Could you check a few things on this model? Use its own coordinates, in mm. Give positions to 0.01 mm unless a question says otherwise; leave off trailing zeros. Loops run counter-clockwise (first coordinate to the right, second up) from the corner with the lowest first, then second, coordinate; pieces in that order, holes last.
1. Imagine slicing it at A-A (x = 0). List the corners of the cut face in (y, z) for me (3 decimals).
2. I need wall thicknesses on line 1 along X through (y, z) = (1.75, -21.5); line 2 along Z through (x, y) = (0, 2.9) (3 decimals); line 3 along Z through (x, y) = (11, 2). Which ranges of each line are inside material? Lowest first, please.
3. Thinking about a two-plate mould opening in Z: for faces 1 (the flat face through (0, 3.81, 14)), 2 (the cylindrical face through (-25.7, 2.425, 19.706)), 3 (the cylindrical face through (14.264, 1.932, -19.645)), which applies, +Z half, -Z half, draft (parallel to the pull), parting line (faces both ways), or undercut?
4. For P1, Ø15.5, axis at x = 0, z = 0, coming from the +Y side; P2, Ø1, axis at x = -1.5, y = 0.5, coming from the -Z side; P3, Ø1, axis at y = 3.5, z = 12.5, coming from the -X side; P4, Ø1.5, axis at x = -8, y = 3, coming from the +Z side, each with a flat end and sliding along its axis, tell me the tip position at first contact or that it passes through.
5. Imagine slicing it at B-B (z = 0). List the corners of the cut face in (x, y) for me (3 decimals).
6. Imagine slicing it at C-C (y = 3.15). List the corners of the cut face in (x, z) for me (1 decimal), plus the area to 3 significant figures.
```python
from build123d import *

# Parameters (mm, degrees)
SKETCH1_W                      = 32.385
SKETCH1_H                      = 3.81
F_7_0_201_DIAMETER_HOLE1_D     = 5.1054
F_7_0_201_DIAMETER_HOLE1_DEPTH = 3.81
HOLE1_D                        = 25.654
HOLE1_DEPTH                    = 3.81
FILLET1_R                      = 1


with BuildPart() as part:
    # Sketch1 → Revolve1 (revolve)
    with BuildSketch(Plane(origin=(0, 0, 0), x_dir=(-1, 0, 0), z_dir=(0, 0, -1))):
        with Locations((-16.1925, 1.905)):
            Rectangle(SKETCH1_W, SKETCH1_H)
    revolve(axis=Axis((0, 0, 0), (0, 1, 0)))

    # #7 (0.201) Diameter Hole1
    with Locations(Plane(origin=(0, 0, 0), x_dir=(-1, 0, 0), z_dir=(0, -1, 0))):
        with Locations((11.90625, 20.622229928), (-11.90625, 20.622229928), (-23.8125, 0), (-11.90625, -20.622229928), (11.90625, -20.622229928), (23.8125, 0)):
            Hole(F_7_0_201_DIAMETER_HOLE1_D / 2, depth=F_7_0_201_DIAMETER_HOLE1_DEPTH)

    # Hole1
    with Locations(Plane(origin=(0, 0, 0), x_dir=(-1, 0, 0), z_dir=(0, -1, 0))):
        with Locations((0, 0)):
            Hole(HOLE1_D / 2, depth=HOLE1_DEPTH)

    # Fillet1
    fillet1_edges = [part.edges().sort_by_distance(p)[0] for p in [
        (-32.385, 0, 0),
    ]]
    fillet(fillet1_edges, radius=FILLET1_R)


solid = part.part
```
Derived:
1. outline: (0, -31.385) arc R1 ccw to (1, -32.385) - (3.81, -32.385) - (3.81, -12.827) - (0, -12.827) - close; (0, 12.827) - (3.81, 12.827) - (3.81, 32.385) - (1, 32.385) arc R1 ccw to (0, 31.385) - close
2. line 1: x = -24.22 to -14.3, -9.51 to 9.51, 14.3 to 24.22
2. line 2: z = -32.385 to -12.827, 12.827 to 32.385
2. line 3: z = -30.46 to -23.01, -18.24 to -6.6, 6.6 to 18.24, 23.01 to 30.46
3. face 1: draft
3. face 2: parting line
3. face 3: undercut
4. P1: passes through
4. P2: stops at z = -32.36
4. P3: stops at x = -30.08
4. P4: stops at z = 31.56
5. outline: (-32.385, 1) arc R1 ccw to (-31.385, 0) - (-26.365, 0) - (-26.365, 3.81) - (-32.385, 3.81) - close; (-21.26, 0) - (-12.827, 0) - (-12.827, 3.81) - (-21.26, 3.81) - close; (12.827, 0) - (21.26, 0) - (21.26, 3.81) - (12.827, 3.81) - close; (26.365, 0) - (31.385, 0) arc R1 ccw to (32.385, 1) - (32.385, 3.81) - (26.365, 3.81) - close
6. outline: circle Ø64.8 at (0, 0); hole circle Ø5.1 at (-23.8, 0); hole circle Ø5.1 at (-11.9, -20.6); hole circle Ø5.1 at (-11.9, 20.6); hole circle Ø25.7 at (0, 0); hole circle Ø5.1 at (11.9, -20.6); hole circle Ø5.1 at (11.9, 20.6); hole circle Ø5.1 at (23.8, 0)
6. area: 2,660 mm2
